from build123d import *

# Parameters (mm, degrees)
SKETCH_1_R          = 2.1
EXTRUDE_1_DEPTH     = 5
EXTRUDE_2_DEPTH     = 5
EXTRUDE_3_DEPTH     = 10
SKETCH_4_R          = 2.1
CUT_EXTRUDE_1_DEPTH = 10
SKETCH_5_R          = 2.1
CUT_EXTRUDE_2_DEPTH = 157.444761979
CUT_EXTRUDE_3_DEPTH = 6
EXTRUDE_4_DEPTH     = 64.5
EXTRUDE_5_DEPTH     = 4
SKETCH_9_W          = 49.5
SKETCH_9_H          = 57.77011897
EXTRUDE_6_DEPTH     = 10
SKETCH_10_W         = 5
SKETCH_10_H         = 48.77011897
CUT_EXTRUDE_4_DEPTH = 10
CUT_EXTRUDE_5_REACH = 172.895
SKETCH_11_R         = 2.5629981
SKETCH_11_R_2       = 2.780591795
FILLET_1_R          = 2
SKETCH_12_R         = 2.1
CUT_EXTRUDE_6_DEPTH = 10
SKETCH_13_W         = 8
SKETCH_13_H         = 48.77011897
CUT_EXTRUDE_7_DEPTH = 5


with BuildPart() as part:
    # 草圖1 → 填料-伸長1 (new body)
    # profile 1 of 2: a face of its own
    with BuildSketch(Plane.XY):
        Polygon((46.554726499, 40.372196633), (35.007721115, 40.372196633), (59.841223807, -2.64069176), (65.614726499, 7.35930824), align=None)
        with Locations((56.75459948, 12.705498399)):
            Circle(SKETCH_1_R, mode=Mode.SUBTRACT)
        with Locations((46.75459948, 30.026006474)):
            Circle(SKETCH_1_R, mode=Mode.SUBTRACT)
    # profile 2 of 2: a face of its own
    with BuildSketch(Plane.XY):
        Polygon((54.456814697, 40.372196633), (46.554726499, 40.372196633), (65.614726499, 7.35930824), (69.565770598, 14.202717363), align=None)
    extrude(amount=EXTRUDE_1_DEPTH)

    # 草圖2 → 填料-伸長2 (add)
    with BuildSketch(Plane.XY.offset(5)):
        Polygon((54.456814697, 40.372196633), (69.565770598, 14.202717363), (65.614726499, 7.35930824), (46.554726499, 40.372196633), align=None)
    extrude(amount=EXTRUDE_2_DEPTH)

    # 草圖3 → 填料-伸長3 (add)
    with BuildSketch(Plane(origin=(0, 0, 0), x_dir=(-1, 0, 0), z_dir=(0, 0, -1))):
        Polygon((-69.565770598, 14.202717363), (-112.641874182, -10.667282637), (-123.034179028, -4.667282637), (-64.849119543, 96.112196633), (-54.456814697, 90.112196633), (-54.456814697, 40.372196633), align=None)
    extrude(amount=-EXTRUDE_3_DEPTH)

    # 草圖4 → 除料-伸長1 (cut)
    with BuildSketch(Plane(origin=(0, 0, 0), x_dir=(-1, 0, 0), z_dir=(0, 0, -1))):
        with Locations((-113.495975798, -4.146630029)):
            Circle(SKETCH_4_R)
        with Locations((-105.495975798, 9.709776431)):
            Circle(SKETCH_4_R)
    extrude(amount=-CUT_EXTRUDE_1_DEPTH, mode=Mode.SUBTRACT)

    # 草圖5 → 除料-伸長2 (cut, through all)
    with BuildSketch(Plane(origin=(0, 0, 0), x_dir=(-1, 0, 0), z_dir=(0, 0, -1))):
        with Locations((-60.530916312, 87.591544025)):
            Circle(SKETCH_5_R)
        with Locations((-68.530916312, 73.735137564)):
            Circle(SKETCH_5_R)
    extrude(amount=-CUT_EXTRUDE_2_DEPTH, mode=Mode.SUBTRACT)

    # 草圖6 → 除料-伸長3 (cut)
    with BuildSketch(Plane.XY.offset(10)):
        Polygon((79.499119543, 70.737652302), (54.456814697, 56.279470858), (54.456814697, 90.112196633), (64.849119543, 96.112196633), align=None)
        Polygon((83.341874182, 6.24908025), (108.384179028, 20.707261694), (123.034179028, -4.667282637), (112.641874182, -10.667282637), align=None)
    extrude(amount=-CUT_EXTRUDE_3_DEPTH, mode=Mode.SUBTRACT)

    # 草圖7 → 填料-伸長4 (add)
    with BuildSketch(Plane.XY.offset(10)):
        Polygon((78.841874182, 8.847156461), (106.134179028, 24.604376011), (108.384179028, 20.707261694), (83.341874182, 6.24908025), align=None)
        Polygon((54.456814697, 56.279470858), (79.499119543, 70.737652302), (81.749119543, 66.840537985), (54.456814697, 51.083318435), align=None)
    extrude(amount=EXTRUDE_4_DEPTH)

    # 草圖8 → 填料-伸長5 (add)
    with BuildSketch(Plane.XY.offset(74.5)):
        Polygon((79.499119543, 70.737652302), (108.384179028, 20.707261694), (83.341874182, 6.24908025), (69.565770598, 14.202717363), (65.614726499, 7.35930824), (46.554726499, 40.372196633), (54.456814697, 40.372196633), (54.456814697, 56.279470858), align=None)
    extrude(amount=-EXTRUDE_5_DEPTH)

    # 草圖9 → 填料-伸長6 (add)
    with BuildSketch(Plane(origin=(90.254641606, 52.108541627, 0), x_dir=(0, 0, -1), z_dir=(0.8660254037844403, 0.4999999999999973, 0))):
        with Locations((-49.75, -7.374015359)):
            Rectangle(SKETCH_9_W, SKETCH_9_H)
    extrude(amount=-EXTRUDE_6_DEPTH)

    # 草圖10 → 除料-伸長4 (cut)
    with BuildSketch(Plane(origin=(90.254641606, 52.108541627, 0), x_dir=(0, 0, -1), z_dir=(0.8660254037844403, 0.4999999999999973, 0))):
        with Locations((-2.5, -7.374015359)):
            Rectangle(SKETCH_10_W, SKETCH_10_H)
    extrude(amount=-CUT_EXTRUDE_4_DEPTH, mode=Mode.SUBTRACT)

    # 草圖11 → 除料-伸長5 (cut, up to next)
    with BuildSketch(Plane(origin=(0, 0, 5), x_dir=(-1, 0, 0), z_dir=(0, 0, -1)), mode=Mode.PRIVATE) as cut_extrude_5_sk1:
        with Locations(Location((-96.496872332, 32.896680856, 0), (0, 0, 90))):
            Circle(SKETCH_11_R)
    cut_extrude_5_tool1 = extrude(cut_extrude_5_sk1.sketch, amount=-CUT_EXTRUDE_5_REACH, mode=Mode.PRIVATE) & part.part
    # 草圖11 → 除料-伸長5 (cut, up to next)
    with BuildSketch(Plane(origin=(0, 0, 5), x_dir=(-1, 0, 0), z_dir=(0, 0, -1)), mode=Mode.PRIVATE) as cut_extrude_5_sk2:
        with Locations(Location((-84.111812847, 54.348233139, 0), (0, 0, 90))):
            Circle(SKETCH_11_R_2)
    cut_extrude_5_tool2 = extrude(cut_extrude_5_sk2.sketch, amount=-CUT_EXTRUDE_5_REACH, mode=Mode.PRIVATE) & part.part
    add(cut_extrude_5_tool1.solids().sort_by_distance((96.496872, 32.896681, 5))[0], mode=Mode.SUBTRACT)
    add(cut_extrude_5_tool2.solids().sort_by_distance((84.111813, 54.348233, 5))[0], mode=Mode.SUBTRACT)

    # 圓角1
    fillet_1_edges = [part.edges().sort_by_distance(p)[0] for p in [
        (93.941649285, 45.722456998, 74.5),
        (114.584179028, 9.968546687, 0),
        (73.299119543, 81.476367309, 0),
    ]]
    fillet(fillet_1_edges, radius=FILLET_1_R)

    # 草圖12 → 除料-伸長6 (cut)
    with BuildSketch(Plane(origin=(90.254641606, 52.108541627, 0), x_dir=(0, 0, -1), z_dir=(0.8660254037844403, 0.4999999999999973, 0))):
        with Locations(Location((-29, -19.759074844, 0), (0, 0, 90))):
            Circle(SKETCH_12_R)
        with Locations(Location((-29, 5.011044126, 0), (0, 0, 90))):
            Circle(SKETCH_12_R)
    extrude(amount=-CUT_EXTRUDE_6_DEPTH, mode=Mode.SUBTRACT)

    # 草圖13 → 除料-伸長7 (cut)
    with BuildSketch(Plane(origin=(90.254641606, 52.108541627, 0), x_dir=(0, 0, -1), z_dir=(0.8660254037844403, 0.4999999999999973, 0))):
        with Locations((-29, -7.374015359)):
            Rectangle(SKETCH_13_W, SKETCH_13_H)
    extrude(amount=-CUT_EXTRUDE_7_DEPTH, mode=Mode.SUBTRACT)


solid = part.part
Here's how the part is built. I have some questions about the finished solid (model axes, mm). A direction names the side the tool comes from. Round coordinates to 2 decimals unless told otherwise and drop trailing zeros. Write each loop counter-clockwise with the first axis right and the second up, starting at its lowest first coordinate (ties: lowest second). Pieces come first, ordered by that corner, then holes.
1. Suppose I cut it at C-C (z = 50). List the corners of the cut face in (x, y) for me, and give its area (3 significant figures).
2. If we mould it in two halves opening along X, with no side actions, what happens to faces 1 (the flat face through (75, 35, 0)), 2 (the flat face through (96.04, 13.58, 38.76)), 3 (the flat face through (101.865, 22.139, 2.535))? For each: released by +X, released by -X, zero draft, split by the parting line, or undercut.
3. Suppose I cut it at A-A (z = 21.5). List the corners of the cut face in (x, y) for me, and give its area (3 significant figures).
4. Suppose I cut it at B-B (x = 51). List the corners of the cut face in (y, z) for me, and give its area (3 significant figures).
5. Will these pins go through, and if not, where does the flat tip stop? pin 1 Ø12 at (x, y) = (53, 7.5) entering from -Z; pin 2 Ø3 at (y, z) = (67.5, 34) entering from +X; pin 3 Ø7.5 at (x, y) = (63.5, 76.5) entering from +Z; pin 4 Ø12 at (y, z) = (26, 45) entering from +X.
6. For faces 4 (the flat face through (67.6, 10.8, 72.5)), 5 (the flat face through (47, 40.372, 4)), 6 (the flat face through (64, 76, 4)), which set-ups out of +Z, -Z, +X, -X, +Y, -Y let a thin tool reach every point of the face, with its end or its side?
7. I need wall thicknesses on L1, parallel to Z at x = 70, y = 16.5; L2, parallel to Z at x = 90, y = 47; L3, parallel to Z at x = 68, y = 78.5. Which ranges of each line are inside material? Lowest first, please.
Answer sheet:
1. outline: (54.46, 51.08) - (73.09, 61.84) - (97.47, 19.6) - (78.84, 8.85) - (83.34, 6.25) - (108.38, 20.71) - (79.5, 70.74) - (54.46, 56.28) - close
1. area: 760 mm2
2. face 1: zero draft
2. face 2: released by +X
2. face 3: undercut
3. outline: (54.46, 51.08) - (81.75, 66.84) - (79.5, 70.74) - (54.46, 56.28) - close; (78.84, 8.85) - (83.34, 6.25) - (108.38, 20.71) - (106.13, 24.6) - close
3. area: 272 mm2
4. outline: (12.67, 0) - (40.37, 0) - (40.37, 10) - (32.67, 10) - (32.67, 5) - (12.67, 5) - close; (32.67, 70.5) - (40.37, 70.5) - (40.37, 74.5) - (32.67, 74.5) - close
4. area: 208 mm2
5. pin 1: stops at z = 0
5. pin 2: stops at x = 82.23
5. pin 3: stops at z = 4
5. pin 4: stops at x = 108.38
6. face 4: +Z, -Z, -Y
6. face 5: +Z, -Z, -X, +Y
6. face 6: +Z, -X, +Y
7. L1: z = 0 to 10, 70.5 to 74.5
7. L2: z = 5 to 10, 33 to 74.5
7. L3: z = 0 to 4
